from build123d import *

# Parameters (mm, degrees)
ESQUISSE15_W             = 32
ESQUISSE15_H             = 20
BOSS_EXTRU_1_DEPTH       = 10
ESQUISSE16_W             = 32
ESQUISSE16_H             = 18
ESQUISSE16_W_2           = 24
ESQUISSE16_H_2           = 13
BOSS_EXTRU_2_DEPTH       = 15
ESQUISSE17_W             = 25
ESQUISSE17_H             = 6
ENL_V_MAT_EXTRU_8_DEPTH  = 4
ESQUISSE19_R             = 1.05
ENL_V_MAT_EXTRU_10_DEPTH = 6
ESQUISSE20_R             = 1.5
ENL_V_MAT_EXTRU_11_DEPTH = 20


with BuildPart() as part:
    # Esquisse15 → Boss.-Extru.1 (new body)
    with BuildSketch(Plane.XY):
        Rectangle(ESQUISSE15_W, ESQUISSE15_H)
    extrude(amount=BOSS_EXTRU_1_DEPTH)

    # Esquisse16 → Boss.-Extru.2 (add)
    with BuildSketch(Plane.XY.offset(10)):
        Rectangle(ESQUISSE16_W, ESQUISSE16_H)
        Rectangle(ESQUISSE16_W_2, ESQUISSE16_H_2, mode=Mode.SUBTRACT)
    extrude(amount=BOSS_EXTRU_2_DEPTH)

    # Esquisse17 → Enlèv. mat.-Extru.8 (cut)
    with BuildSketch(Plane.ZY.offset(16)):
        with Locations((12.5, 0)):
            Rectangle(ESQUISSE17_W, ESQUISSE17_H)
    extrude(amount=-ENL_V_MAT_EXTRU_8_DEPTH, mode=Mode.SUBTRACT)

    # Esquisse19 → Enlèv. mat.-Extru.10 (cut)
    with BuildSketch(Plane.XY.offset(25)):
        with Locations((13.9, 0)):
            Circle(ESQUISSE19_R)
    extrude(amount=-ENL_V_MAT_EXTRU_10_DEPTH, mode=Mode.SUBTRACT)

    # Esquisse20 → Enlèv. mat.-Extru.11 (cut)
    with BuildSketch(Plane(origin=(16, 0, 0), x_dir=(0, 0, -1), z_dir=(1, 0, 0))):
        with Locations((-5, 6)):
            Circle(ESQUISSE20_R)
        with Locations((-5, -6)):
            Circle(ESQUISSE20_R)
    extrude(amount=-ENL_V_MAT_EXTRU_11_DEPTH, mode=Mode.SUBTRACT)


solid = part.part
Could you check a few things on this model? Use its own coordinates, in mm. A direction names the side the tool comes from. Give positions to 0.01 mm unless a question says otherwise; leave off trailing zeros. Write each loop counter-clockwise with the first axis right and the second up, starting at its lowest first coordinate (ties: lowest second). Pieces come first, ordered by that corner, then holes. Notation, with made-up numbers: (-31.5, -40) - (-8.5, -40) arc R27 cw to (-8.5, -10) - close; hole circle Ø6 at (49, 67). An arc over 180 degrees is marked (long way). Use CSV: the item, a comma, the result in double quotes. Start each with the question number.
Item 1: I want a section at C-C, the plane y = 2. Please give me the cut outline in (x, z), then the cut area to 3 significant figures.
Item 2: If we mould it in two halves opening along Y, with no side actions, what happens to faces 1 (the face through (-16, -7, 12)), 2 (the face through (12, 0, 17)), 3 (the face through (0, -9, 17))? For each: pulls with the +Y half, pulls with the -Y half, needs draft (parallel to the pull), parting line crosses it, or undercut.
Item 3: If I drill on line 1 along X through (y, z) = (3.5, 14.75); line 2 along Y through (x, z) = (8.5, 20.25); line 3 along Y through (x, z) = (12.5, 5.25), over which ranges is the centre line in solid material (lowest first)?
Item 4: For faces 4 (the face through (-12, 0, 5)), 5 (the face through (14, 0, 19)), 6 (the face through (-4, -6, 5)), which set-ups out of +Z, -Z, +X, -X, +Y, -Y let a thin tool reach every point of the face, with its end or its side?
Item 5: I want a section at D-D, the plane x = -9. Please give me the cut outline in (y, z), then the cut area to 3 significant figures.
Item 6: I'm going to push flat-ended pins straight in: pin 1 (1.8 mm diameter, centred on y = -1, z = 5, fed in from -X); pin 2 (7.5 mm diameter, centred on x = 1, z = 17.5, fed in from +Y); pin 3 (1 mm diameter, centred on x = -11, z = 11, fed in from -Y). Where does each tip first touch, or does it pass through?
Item 7: I want a section at B-B, the plane z = 15.25. Please give me the cut outline in (x, y), then the cut area to 3 significant figures.
Item 8: I want a section at A-A, the plane x = -1.5. Please give me the cut outline in (y, z).
Findings:
1,outline,"(-12, 0) - (16, 0) - (16, 25) - (12, 25) - (12, 10) - (-12, 10) - close"
1,area,"340 mm2"
2,face 1,"needs draft"
2,face 2,"undercut"
2,face 3,"pulls with the -Y half"
3,line 1,"x = -16 to -12, 12 to 16"
3,line 2,"y = -9 to -6.5, 6.5 to 9"
3,line 3,"y = -10 to -7.48, -4.52 to 4.52, 7.48 to 10"
4,face 4,"+Z, -Z, -X"
4,face 5,"+Z"
4,face 6,"+X"
5,outline,"(-10, 0) - (10, 0) - (10, 10) - (9, 10) - (9, 25) - (6.5, 25) - (6.5, 10) - (-6.5, 10) - (-6.5, 25) - (-9, 25) - (-9, 10) - (-10, 10) - close"
5,area,"275 mm2"
6,pin 1,"stops at x = -12"
6,pin 2,"stops at y = 9"
6,pin 3,"stops at y = -9"
7,outline,"(-16, -9) - (16, -9) - (16, 9) - (-16, 9) - (-16, 3) - (-12, 3) - (-12, 6.5) - (12, 6.5) - (12, -6.5) - (-12, -6.5) - (-12, -3) - (-16, -3) - close"
7,area,"240 mm2"
8,outline,"(-10, 0) - (10, 0) - (10, 10) - (9, 10) - (9, 25) - (6.5, 25) - (6.5, 10) - (-6.5, 10) - (-6.5, 25) - (-9, 25) - (-9, 10) - (-10, 10) - close; hole circle Ø3 at (-6, 5); hole circle Ø3 at (6, 5)"
